Answer from the drawing. Dimensions are ordinates in mm from the lowest x, y and z of the part. Coordinates: 2 decimals unless noted, no trailing zeros. Loops run counter-clockwise (first coordinate to the right, second up) from the corner with the lowest first, then second, coordinate; pieces in that order, holes last. Notation, with made-up numbers: M 17,70.25 L 47,70.25 A21 cw 47,103.25 Z; hole C -40,40.5 d7. An arc over 180 degrees is marked long. One line per item, written item: value. Start each with the question number.
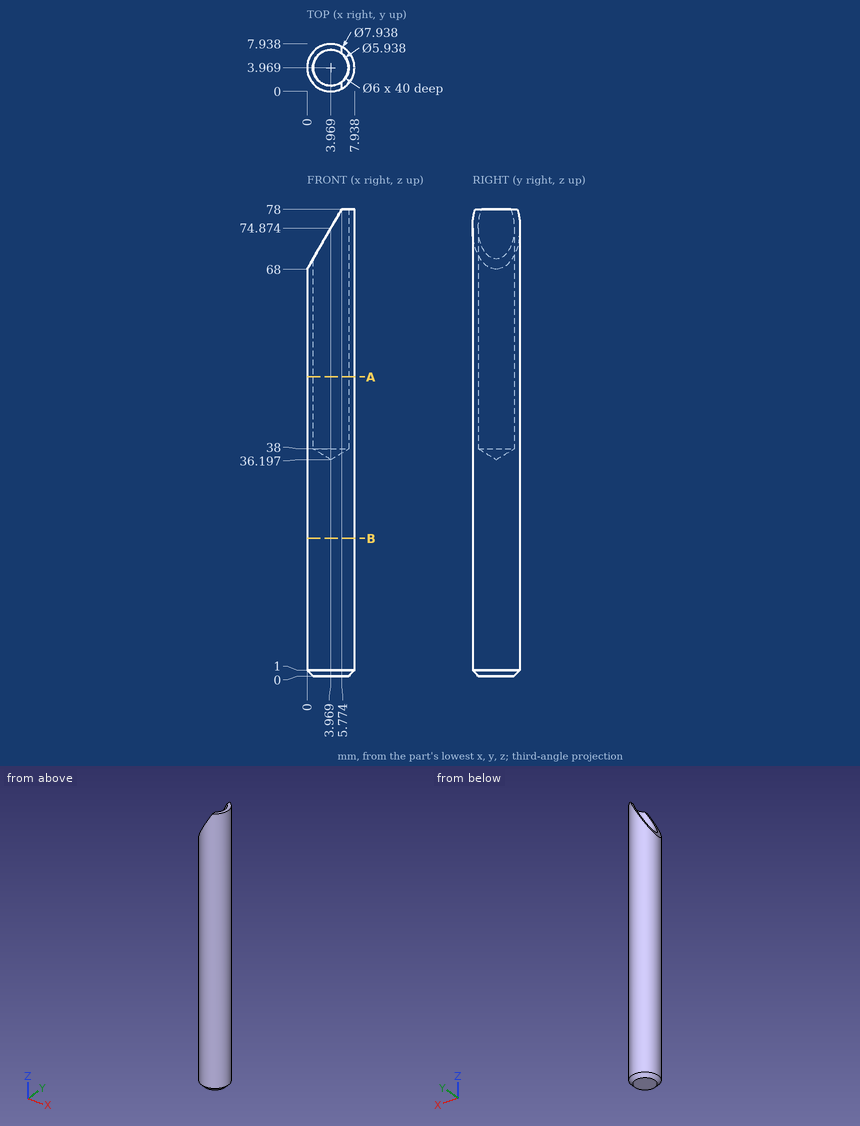
1) Section A-A (z = 50) is taken. Determine the outline of the cut face in (x, y).
2) Section B-B (z = 23) is taken. Determine the outline of the cut face in (x, y).
3) Consider line 1 along Y through (x, z) = (4, 66); line 2 along Y through (x, z) = (3.75, 5). Determine where each line is inside the solid, lowest interval first.
4) Flat-ended cylindrical pins translate along their axes: pin 1 (3 mm diameter, centred on x = 6, z = 41, fed in from +Y); pin 2 (1.5 mm diameter, centred on x = 6, z = 54.5, fed in from +Y) (1 decimal); pin 3 (1.5 mm diameter, centred on y = 5.5, z = 42.5, fed in from +X). Find the tip coordinate at first contact, or state that the pin passes through.
Results found:
1. outline: C 3.97,3.97 d7.94; hole C 3.97,3.97 d6
2. outline: C 3.97,3.97 d7.94
3. line 1: y = 0 to 0.97, 6.97 to 7.94
3. line 2: y = 0.01 to 7.93
4. pin 1: stops at y = 7.9
4. pin 2: stops at y = 7.7
4. pin 3: stops at x = 7.86
